For this review, take the finished solid that the model builds, in its own axes (mm). Face numbers are marked on the shaded views. A direction names the side the tool comes from. Round coordinates to 2 decimals unless told otherwise and drop trailing zeros. Write each loop counter-clockwise with the first axis right and the second up, starting at its lowest first coordinate (ties: lowest second). Pieces come first, ordered by that corner, then holes. Notation, with made-up numbers: (42.5, -5) - (78.5, -5) arc R4 cw to (78.5, 2) - close; hole circle Ø7 at (-20, -37). An arc over 180 degrees is marked (long way). Answer in a Markdown table with one row per item. Add a question column.
from build123d import *

# Parameters (mm, degrees)
F0_R     = 6.35
F1_DEPTH = 12.7
F2_SIZE  = 1.5


with BuildPart() as f1:
    # F0 (on Front) → F1 (new body)
    with BuildSketch(Plane.XZ):
        with BuildLine():
            Line((-70, 20), (-70, 5))
            ThreePointArc((-70, 5), (-68.535534, 1.464466), (-65, 0))
            Line((-65, 0), (12.7, 0))
            Line((12.7, 0), (12.7, 40))
            Line((12.7, 40), (0, 40))
            Line((0, 40), (0, 70))
            Line((0, 70), (-10, 70))
            Line((-10, 70), (-55, 25))
            Line((-55, 25), (-65, 25))
            ThreePointArc((-65, 25), (-68.535534, 23.535534), (-70, 20))
        make_face()
        with Locations((-60, 12.5)):
            Circle(F0_R, mode=Mode.SUBTRACT)
    extrude(amount=F1_DEPTH)

    # F2
    f2_edges = [f1.edges().sort_by_distance(p)[0] for p in [
        (-66.35, 0, 12.5),
        (-66.35, -12.7, 12.5),
    ]]
    chamfer(f2_edges, length=F2_SIZE)


solid = f1.part
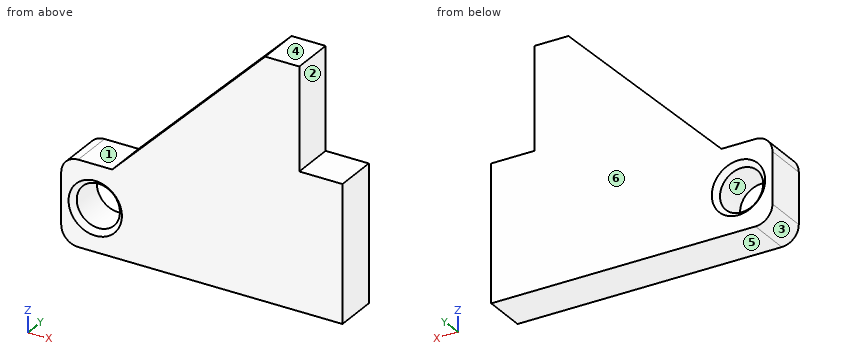
Q1. Add section D-D on z = 62. State the section outline as (x, y) points.
Q2. Draft analysis for pull direction Z (two halves, no side actions). For the marked faces 4, 5, 6 and 7, state which applies: released by +Z, released by -Z, zero draft, split by the parting line, or undercut.
Q3. To check wall thickness, follow probe 1 along Z at (x, y) = (-60, -3.25); probe 2 along Z at (x, y) = (6, -4.5); probe 3 along Z at (x, y) = (-46.5, -7.25). State the ranges of each line that lie inside material, in increasing order.
Q4. Insertion check: pin 1 Ø1.5 at (x, y) = (-29, -10) entering from +Z; pin 2 Ø6.5 at (y, z) = (-9, 58) entering from +X; pin 3 Ø6.5 at (x, y) = (5.5, -6.5) entering from +Z. Each pin has a flat end and moves straight along its axis. Give the tip position at first contact, or say it passes through.
Q5. Add section A-A on z = 12.5. State the section outline as (x, y) points.
Q6. Add section B-B on y = -2.5. State the section outline as (x, z) points, then the cut area to 3 significant figures.
Q7. Add section C-C on x = -60. State the section outline as (y, z) points, then the cut area to 3 significant figures.
Q8. Tool access review of the marked faces 1, 2 and 3: name each direction out of +Z, -Z, +X, -X, +Y, -Y from which nothing blocks a thin tool from reaching the whole face with its end or side.
Answer sheet:
| question | item | result |
|---|---|---|
| 1 | outline | (-18, -12.7) - (0, -12.7) - (0, 0) - (-18, 0) - close |
| 2 | face 4 | released by +Z |
| 2 | face 5 | released by -Z |
| 2 | face 6 | zero draft |
| 2 | face 7 | undercut |
| 3 | probe 1 | z = 0 to 6.15, 18.85 to 25 |
| 3 | probe 2 | z = 0 to 40 |
| 3 | probe 3 | z = 0 to 33.5 |
| 4 | pin 1 | stops at z = 51.75 |
| 4 | pin 2 | stops at x = 0 |
| 4 | pin 3 | stops at z = 40 |
| 5 | outline | (-70, -12.7) - (-67.85, -12.7) - (-66.35, -11.2) - (-66.35, -1.5) - (-67.85, 0) - (-70, 0) - close; (-53.65, -11.2) - (-52.15, -12.7) - (12.7, -12.7) - (12.7, 0) - (-52.15, 0) - (-53.65, -1.5) - close |
| 6 | outline | (-70, 5) arc R5 ccw to (-65, 0) - (12.7, 0) - (12.7, 40) - (0, 40) - (0, 70) - (-10, 70) - (-55, 25) - (-65, 25) arc R5 ccw to (-70, 20) - close; hole circle Ø12.7 at (-60, 12.5) |
| 6 | area | 3,580 mm² |
| 7 | outline | (-12.7, 0) - (0, 0) - (0, 4.65) - (-1.5, 6.15) - (-11.2, 6.15) - (-12.7, 4.65) - close; (-12.7, 20.35) - (-11.2, 18.85) - (-1.5, 18.85) - (0, 20.35) - (0, 25) - (-12.7, 25) - close |
| 7 | area | 152 mm² |
| 8 | face 1 | +Z, -X, +Y, -Y |
| 8 | face 2 | +Z, +X, +Y, -Y |
| 8 | face 3 | -Z, -X, +Y, -Y |
